```python
from build123d import *

# Parameters (mm, degrees)
SKETCH_1_R            = 55
EXTRUDE_1_DEPTH       = 5
SKETCH_2_R            = 49.9
EXTRUDE_2_DEPTH       = 5
SKETCH_3_W            = 35
SKETCH_3_H            = 45
EXTRUDE_3_DEPTH       = 25
SKETCH_4_W            = 20.2
SKETCH_4_H            = 10.3
CUT_EXTRUDE_1_DEPTH   = 78.5
SKETCH_5_R            = 4.1
CUT_EXTRUDE_2_DEPTH   = 11
SKETCH_6_R            = 2.75
CUT_EXTRUDE_3_DEPTH   = 36
CHAMFER1_SIZE         = 2
CHAMFER1_SIZE2        = 0.535898385
CHAMFER1_PART_2_SIZE  = 2
CHAMFER1_PART_2_SIZE2 = 0.535898385
CHAMFER1_PART_3_SIZE  = 2
CHAMFER1_PART_3_SIZE2 = 0.535898385
CHAMFER1_PART_4_SIZE  = 2
CHAMFER1_PART_4_SIZE2 = 0.535898385
SKETCH2_W             = 35.065209797
SKETCH2_H             = 45
CUT_EXTRUDE1_DEPTH    = 12.5
BOSS_EXTRUDE1_START   = -2
SKETCH4_W             = 70
SKETCH4_H             = 45
BOSS_EXTRUDE1_DEPTH   = 5.35
SKETCH5_R             = 4.15
CUT_EXTRUDE2_DEPTH    = 16.3500001
CUT_EXTRUDE3_DEPTH    = 6.5
SKETCH7_W             = 20
SKETCH7_H             = 34
CUT_EXTRUDE4_DEPTH    = 5
CHAMFER2_SIZE         = 1
CHAMFER2_SIZE2        = 2.747477419


with BuildPart() as part:
    # Эскиз1 → Бобышка-Вытянуть1 (new body)
    with BuildSketch(Plane(origin=(0, 0, 0), x_dir=(1, 0, 0), z_dir=(0, 1, 0))):
        Circle(SKETCH_1_R)
    extrude(amount=EXTRUDE_1_DEPTH)

    # Эскиз2 → Бобышка-Вытянуть2 (add)
    with BuildSketch(Plane(origin=(0, 5, 0), x_dir=(1, 0, 0), z_dir=(0, 1, 0))):
        Circle(SKETCH_2_R)
    extrude(amount=EXTRUDE_2_DEPTH)

    # Эскиз3 → Бобышка-Вытянуть3 (add)
    with BuildSketch(Plane.XZ):
        Rectangle(SKETCH_3_W, SKETCH_3_H)
    extrude(amount=EXTRUDE_3_DEPTH)

    # Эскиз4 → Вырез-Вытянуть1 (cut, through all)
    with BuildSketch(Plane.XY.offset(22.5)):
        with Locations((0, -12.5)):
            Rectangle(SKETCH_4_W, SKETCH_4_H)
    extrude(amount=-CUT_EXTRUDE_1_DEPTH, mode=Mode.SUBTRACT)

    # Эскиз5 → Вырез-Вытянуть2 (cut, through all)
    with BuildSketch(Plane.XZ):
        with Locations((33.592198598, -32.871936263)):
            Circle(SKETCH_5_R)
        with Locations((-33.591727056, -32.872418125)):
            Circle(SKETCH_5_R)
        with Locations((-33.591727056, 32.872418125)):
            Circle(SKETCH_5_R)
        with Locations((33.483215177, 32.983215177)):
            Circle(SKETCH_5_R)
    extrude(amount=-CUT_EXTRUDE_2_DEPTH, mode=Mode.SUBTRACT)

    # Эскиз6 → Вырез-Вытянуть3 (cut, through all)
    with BuildSketch(Plane(origin=(0, 10, 0), x_dir=(1, 0, 0), z_dir=(0, 1, 0))):
        with Locations((-17.999799176, 27.999999999)):
            Circle(SKETCH_6_R)
    extrude(amount=-CUT_EXTRUDE_3_DEPTH, mode=Mode.SUBTRACT)

    # Chamfer1
    chamfer1_edges = [part.edges().sort_by_distance(p)[0] for p in [
        (0.000357897, 10, -49.899999999),
    ]]
    chamfer1_side = [part.faces().sort_by_distance(p)[0] for p in [
        (0.000357897, 7.5, -49.899999999),
    ]]
    chamfer(chamfer1_edges, length=CHAMFER1_SIZE, length2=CHAMFER1_SIZE2, reference=chamfer1_side[0])

    # Chamfer1 part 2
    chamfer1_part_2_edges = [part.edges().sort_by_distance(p)[0] for p in [
        (-49.9, 10, 0),
    ]]
    chamfer1_part_2_side = [part.faces().sort_by_distance(p)[0] for p in [
        (-49.9, 7.5, 0),
    ]]
    chamfer(chamfer1_part_2_edges, length=CHAMFER1_PART_2_SIZE, length2=CHAMFER1_PART_2_SIZE2, reference=chamfer1_part_2_side[0])

    # Chamfer1 part 3
    chamfer1_part_3_edges = [part.edges().sort_by_distance(p)[0] for p in [
        (-0.08242255, 10, 49.899931929),
    ]]
    chamfer1_part_3_side = [part.faces().sort_by_distance(p)[0] for p in [
        (-0.08242255, 7.5, 49.899931929),
    ]]
    chamfer(chamfer1_part_3_edges, length=CHAMFER1_PART_3_SIZE, length2=CHAMFER1_PART_3_SIZE2, reference=chamfer1_part_3_side[0])

    # Chamfer1 part 4
    chamfer1_part_4_edges = [part.edges().sort_by_distance(p)[0] for p in [
        (49.899931657, 10, 0.082587101),
    ]]
    chamfer1_part_4_side = [part.faces().sort_by_distance(p)[0] for p in [
        (49.899931657, 7.5, 0.082587101),
    ]]
    chamfer(chamfer1_part_4_edges, length=CHAMFER1_PART_4_SIZE, length2=CHAMFER1_PART_4_SIZE2, reference=chamfer1_part_4_side[0])

    # Sketch2 → Cut-Extrude1 (cut)
    with BuildSketch(Plane.XZ.offset(25)):
        with Locations((-0.032604899, 0)):
            Rectangle(SKETCH2_W, SKETCH2_H)
    extrude(amount=-CUT_EXTRUDE1_DEPTH, mode=Mode.SUBTRACT)

    # Sketch4 → Boss-Extrude1 (add)
    with BuildSketch(Plane.XZ.offset(7.35).offset(BOSS_EXTRUDE1_START)):
        Rectangle(SKETCH4_W, SKETCH4_H)
    extrude(amount=-BOSS_EXTRUDE1_DEPTH)

    # Sketch5 → Cut-Extrude2 (cut, through all)
    with BuildSketch(Plane.XZ.offset(5.35)):
        with Locations((25, 15)):
            Circle(SKETCH5_R)
        with Locations((-25, 15)):
            Circle(SKETCH5_R)
        with Locations((25, -15)):
            Circle(SKETCH5_R)
        with Locations((-25, -15)):
            Circle(SKETCH5_R)
    extrude(amount=-CUT_EXTRUDE2_DEPTH, mode=Mode.SUBTRACT)

    # Sketch6 → Cut-Extrude3 (cut)
    with BuildSketch(Plane(origin=(0, 10, 0), x_dir=(1, 0, 0), z_dir=(0, 1, 0))):
        Polygon((-18.504809472, -11.25), (-25, -7.5), (-31.495190528, -11.25), (-31.495190528, -18.75), (-25, -22.5), (-18.504809472, -18.75), align=None)
        Polygon((31.495190528, -11.25), (25, -7.5), (18.504809472, -11.25), (18.504809472, -18.75), (25, -22.5), (31.495190528, -18.75), align=None)
        Polygon((31.495190528, 18.75), (25, 22.5), (18.504809472, 18.75), (18.504809472, 11.25), (25, 7.5), (31.495190528, 11.25), align=None)
        Polygon((-18.504809472, 18.75), (-25, 22.5), (-31.495190528, 18.75), (-31.495190528, 11.25), (-25, 7.5), (-18.504809472, 11.25), align=None)
    extrude(amount=-CUT_EXTRUDE3_DEPTH, mode=Mode.SUBTRACT)

    # Sketch7 → Cut-Extrude4 (cut)
    with BuildSketch(Plane(origin=(0, 10, 0), x_dir=(1, 0, 0), z_dir=(0, 1, 0))):
        Rectangle(SKETCH7_W, SKETCH7_H)
    extrude(amount=-CUT_EXTRUDE4_DEPTH, mode=Mode.SUBTRACT)

    # Chamfer2
    chamfer2_edges = [part.edges().sort_by_distance(p)[0] for p in [
        (-18.504809472, 10, 15),
        (-21.752404736, 10, 9.375),
        (-28.247595264, 10, 9.375),
        (-31.495190528, 10, 15),
        (-28.247595264, 10, 20.625),
        (-21.752404736, 10, 20.625),
        (31.495190528, 10, 15),
        (28.247595264, 10, 9.375),
        (21.752404736, 10, 9.375),
        (18.504809472, 10, 15),
        (21.752404736, 10, 20.625),
        (28.247595264, 10, 20.625),
        (31.495190528, 10, -15),
        (28.247595264, 10, -20.625),
        (21.752404736, 10, -20.625),
        (18.504809472, 10, -15),
        (21.752404736, 10, -9.375),
        (28.247595264, 10, -9.375),
        (-18.504809472, 10, -15),
        (-21.752404736, 10, -20.625),
        (-28.247595264, 10, -20.625),
        (-31.495190528, 10, -15),
        (-28.247595264, 10, -9.375),
        (-21.752404736, 10, -9.375),
    ]]
    chamfer2_side = [part.faces().sort_by_distance(p)[0] for p in [
        (29.567670169, 10, 29.126140435),
    ]]
    chamfer(chamfer2_edges, length=CHAMFER2_SIZE, length2=CHAMFER2_SIZE2, reference=chamfer2_side[0])


solid = part.part
```
Can you work these out from the model? Positions are in its coordinate system, mm. A direction names the side the tool comes from. Give positions to 0.01 mm unless a question says otherwise; leave off trailing zeros. Loops run counter-clockwise (first coordinate to the right, second up) from the corner with the lowest first, then second, coordinate; pieces in that order, holes last. Notation, with made-up numbers: M 52,46 L 102,46 A16 cw 102,63 Z; hole C 84.5,-30 d3. An arc over 180 degrees is marked long. Use one line per item in the form item = value. Start each with the question number.
(1) I want a section at B-B, the plane z = 13.5. State how many separate pieces and enclosed holes the cut face has, and give its area (3 significant figures).
(2) I want a section at A-A, the plane y = -1.5. Write out the boundary of the cut face in (x, z).
(3) I'm going to push flat-ended pins straight in: P1, Ø1, axis at x = 15, y = -8, coming from the +Z side; P2, Ø2, axis at y = -2.5, z = 42, coming from the -X side; P3, Ø4, axis at x = 1.5, z = -10.5, coming from the -Y side; P4, Ø1.1, axis at y = 6, z = -13.5, coming from the -X side. Where does each tip first touch, or does it pass through?
(4) Please list where these lines run through material, in increasing order: line 1 (Z direction, x = -25, y = -3.5); line 2 (X direction, y = -0.5, z = 16); line 3 (X direction, y = -11, z = -3).
(5) On a 3-axis mill with a long thin cutter (end or side, diameter ignored), from which of +Z, -Z, +X, -X, +Y, -Y can I reach the whole of each face in a straight line? I mean faces 1 (the flat face through (0, -5, 22.5)), 2 (the flat face through (-21.558, 8.607, 21.082)), 3 (the flat face through (-1, 0, 24)). Say none if no direction works.
(6) Thinking about a two-plate mould opening in X: for faces 4 (the flat face through (0, -5, -22.5)), 5 (the flat face through (17.5, -9, 0)), 6 (the cylindrical face through (-31.388, 4.93, -29.415)), which applies, released by +X, released by -X, zero draft, split by the parting line, or undercut?
Worked out:
q1.separate_pieces = 3
q1.enclosed_holes = 0
q1.area = 1,120 mm²
q2.outline = M -35,-22.5 L 35,-22.5 L 35,22.5 L -35,22.5 Z; hole C -25,-15 d8.3; hole C -25,15 d8.3; hole C 25,-15 d8.3; hole C 25,15 d8.3
q3.P1 = 22.5
q3.P2 = through
q3.P3 = -7.35
q3.P4 = -48.19
q4.line_1 = -22.5 to -19.15, -10.85 to 10.85, 19.15 to 22.5
q4.line_2 = -35 to -29.03, -20.97 to 20.97, 29.03 to 35
q4.line_3 = -17.5 to -10.1, 10.1 to 17.5
q5.face_1 = +Z, +X, -X, -Y
q5.face_2 = +Y
q5.face_3 = -Y
q6.face_4 = zero draft
q6.face_5 = released by +X
q6.face_6 = undercut
